For this review, take the finished solid that the model builds, in its own axes (mm). Round coordinates to 2 decimals unless told otherwise and drop trailing zeros. One line per item, written item: value. Start each with the question number.
Q1. Clearance check with flat-ended pins moving along their axes: pin 1 Ø5 at (x, y) = (-40.39, 0) entering from -Z; pin 2 Ø2.5 at (x, y) = (40.39, 0) entering from +Z. State where each tip first meets the part, or that it passes through.
Q2. For probe 1 along X at (y, z) = (5, 0.45); probe 2 along X at (y, z) = (3.75, -0.2); probe 3 along Y at (x, z) = (27, 0.2), list the stretches that pass through material, from the lowest coordinate up.
Q3. Mouldability with a two-part tool opening along Y and no side actions: class faces 1 (the face through (-1, 0, 0.5)), 2 (the face through (38.96, 0.45, -0.01)) as +Y half, -Y half, draft (parallel to the pull), parting line (faces both ways), or undercut.
Q4. Add section A-A on y = 0. Give the number of separate pieces and of enclosed holes in the cut face, and give its area (3 significant figures).
```python
from build123d import *

# Parameters (mm, degrees)
EXTRUDE_1_DEPTH      = 0.5
EXTRUDE_1_DEPTH_BACK = 0.5
SKETCH_1_W           = 100
SKETCH_1_H           = 20
CUT_EXTRUDE_1_DEPTH  = 52
SKETCH_8_R           = 1.5
CUT_EXTRUDE_2_DEPTH  = 52.00000012
SKETCH_9_R           = 1.05
EXTRUDE_2_DEPTH      = 2
OTHER_START          = -2.5
OTHER_2_OUTLINE_R    = 1.05
OTHER_2_DEPTH        = 2


# Read off the part's stored shape, not the designer's step: Пересечение2
with BuildPart() as part:
    # Эскиз1 → Бобышка-Вытянуть1 (new, two sides: drawn at the far end of the back side and taken through both)
    with BuildSketch(Plane.XY.offset(-EXTRUDE_1_DEPTH_BACK)):
        Rectangle(SKETCH_1_W, SKETCH_1_H)
    extrude(amount=EXTRUDE_1_DEPTH + EXTRUDE_1_DEPTH_BACK)

    # Эскиз7 → Вырез-Вытянуть1 (cut, through all)
    with BuildSketch(Plane.XY.offset(0.5)):
        with BuildLine():
            ThreePointArc((37.261495637, 5.33423095), (37.952030231, 4.100066466), (39.186194715, 4.79060106))
            add(Edge.make_bspline(
                [(39.186194715, 4.79060106), (39.206075717, 4.860988923), (39.262496645, 4.988405972), (39.480772307, 5.263607744), (39.972116976, 5.552949613), (40.89012751, 5.611168859), (42.346211172, 5.064723366), (44.026902125, 2.933159087), (43.815557835, -1.408653234), (40.817030581, -4.80884968), (37.021062322, -6.164885186), (33.732157303, -6.253240822), (30.314099065, -5.243442536), (27.144697082, -3.082909818), (25.035720973, -0.378766084), (23.85308145, 2.208270108), (23.449186454, 3.64108751), (23.305322842, 4.359662985)],
                knots=[0, 0, 0, 0, 0.03125, 0.0625, 0.125, 0.1875, 0.25, 0.375, 0.5, 0.625, 0.6875, 0.75, 0.8125, 0.875, 0.9375, 0.96875, 1, 1, 1, 1], degree=3))
            ThreePointArc((23.305322842, 4.359662985), (22.128470162, 5.143893671), (21.344239476, 3.96704099))
            add(Edge.make_bspline(
                [(37.261495637, 5.33423095), (37.539855307, 6.319751815), (39.275153501, 7.946538331), (43.246471825, 7.317604488), (46.129826318, 3.464099405), (45.771597181, -2.30217859), (41.988507816, -6.528062966), (37.380831362, -8.166298308), (33.454677533, -8.267248255), (29.431863805, -7.074452826), (25.746418814, -4.55740521), (23.320064013, -1.441995451), (21.967408891, 1.518598896), (21.5081203, 3.148482776), (21.344239476, 3.96704099)],
                knots=[0, 0, 0, 0, 0.125, 0.25, 0.375, 0.5, 0.625, 0.6875, 0.75, 0.8125, 0.875, 0.9375, 0.96875, 1, 1, 1, 1], degree=3))
        make_face()
    extrude(amount=-CUT_EXTRUDE_1_DEPTH, mode=Mode.SUBTRACT)

    # Эскиз8 → Вырез-Вытянуть2 (cut, through all)
    with BuildSketch(Plane(origin=(0, 0, -0.5), x_dir=(-1, 0, 0), z_dir=(0, 0, -1))):
        with Locations((-40.392058098, 0)):
            Circle(SKETCH_8_R)
    cut_extrude_2 = extrude(amount=-CUT_EXTRUDE_2_DEPTH, mode=Mode.SUBTRACT)

    # Зеркальное отражение1: Вырез-Вытянуть2 across plane
    add(cut_extrude_2.mirror(Plane(origin=(0, 0, 0), x_dir=(0, 0, 1), z_dir=(1, 0, 0))), mode=Mode.SUBTRACT)


with BuildPart() as body_2:
    # Эскиз9 → Бобышка-Вытянуть2 (new body)
    with BuildSketch(Plane(origin=(0, 0, -0.5), x_dir=(-1, 0, 0), z_dir=(0, 0, -1))):
        with BuildLine():
            Line((-38.223845176, 7.062416005), (-136.223845176, 7.062416005))
            Line((-136.223845176, 7.062416005), (-136.223845176, 3.062416005))
            Line((-136.223845176, 3.062416005), (-38.223845176, 3.062416005))
            ThreePointArc((-38.223845176, 3.062416005), (-36.223845176, 5.062416005), (-38.223845176, 7.062416005))
        make_face()
        with Locations((-38.223845176, 5.062416005)):
            Circle(SKETCH_9_R, mode=Mode.SUBTRACT)
    extrude(amount=EXTRUDE_2_DEPTH)

    # Пересечение2 outline → Пересечение2 (cut)
    with BuildSketch(Plane.XY.offset(OTHER_START)):
        with BuildLine():
            Line((136.223845176, 7.062416005), (38.223845176, 7.062416005))
            ThreePointArc((38.223845176, 7.062416005), (36.223845176, 5.062416005), (38.223845176, 3.062416005))
            Line((38.223845176, 3.062416005), (136.223845176, 3.062416005))
            Line((136.223845176, 3.062416005), (136.223845176, 7.062416005))
        make_face()
        with Locations((38.223845176, 5.062416005)):
            Circle(OTHER_2_OUTLINE_R, mode=Mode.SUBTRACT)
    extrude(amount=OTHER_2_DEPTH, mode=Mode.SUBTRACT)


solid = part.part
```
Result set:
1. pin 1: stops at z = -0.5
1. pin 2: passes through
2. probe 1: x = -50 to 21.78, 22.87 to 37.23, 39.28 to 42.12, 44.79 to 50
2. probe 2: x = -50 to 21.39, 23.44 to 43.21, 45.4 to 50
2. probe 3: y = -10 to -5.32, -2.66 to 10
3. face 1: draft
3. face 2: undercut
4. separate pieces: 5
4. enclosed holes: 0
4. area: 89.7 mm^2
